```python
from build123d import *

# Parameters (mm, degrees)
F1_DEPTH = 127
F3_D     = 6.7564
F5_D     = 6.7564


with BuildPart() as f1:
    # F0 (on Front) → F1 (new body)
    with BuildSketch(Plane.XZ):
        Polygon((0, 38.1), (0, 0), (15.875, 0), (15.875, 3.175), (3.175, 3.175), (3.175, 38.1), align=None)
    extrude(amount=F1_DEPTH)

    # F3 (through all)
    with Locations(Plane.YZ.offset(3.175)):
        with Locations((-114.3, 25.4), (-63.5, 25.4), (-12.7, 25.4)):
            Hole(F3_D / 2)

    # F5 (through all)
    with Locations(Plane.XY.offset(3.175)):
        with Locations((9.525, -101.6), (9.525, -25.4), (9.525, -76.2), (9.525, -50.8)):
            Hole(F5_D / 2)


solid = f1.part
```
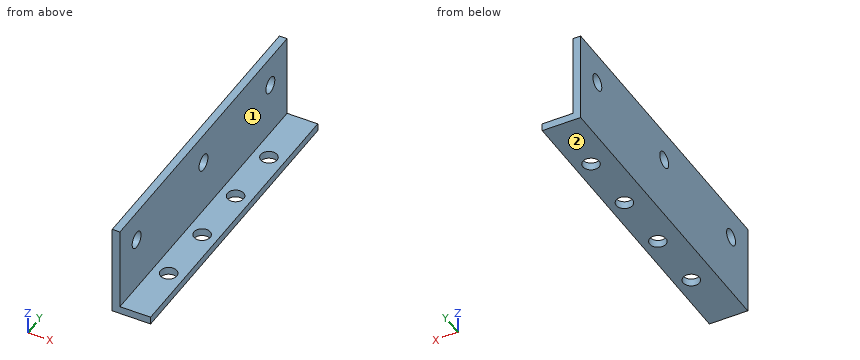
Here's how the part is built. I have some questions about the finished solid (model axes, mm). Face numbers are marked on the shaded views. A direction names the side the tool comes from. Round coordinates to 2 decimals unless told otherwise and drop trailing zeros. Write each loop counter-clockwise with the first axis right and the second up, starting at its lowest first coordinate (ties: lowest second). Pieces come first, ordered by that corner, then holes. Notation, with made-up numbers: M 57,-3.75 L 73,-3.75 A22 ccw 73,15.25 Z; hole C 4.25,-6 d10. An arc over 180 degrees is marked long. Answer as CSV lines item,"result". Start each with the question number.
1. Suppose I cut it at B-B on x = 9. Write out the boundary of the cut face in (y, z) (3 decimals).
2. I need wall thicknesses on probe 1 along Y at (x, z) = (1, 27); probe 2 along Y at (x, z) = (9, 2); probe 3 along Z at (x, y) = (2.1, -114.3). Which ranges of each line are inside material? Lowest first, please.
3. Suppose I cut it at A-A on y = -101.6. Write out the boundary of the cut face in (x, z) (3 decimals).
4. On a 3-axis mill with a long thin cutter (end or side, diameter ignored), from which of +Z, -Z, +X, -X, +Y, -Y can I reach the whole of each face in a straight line? I mean the marked faces 1 and 2. Say none if no direction works.
5. Suppose I cut it at D-D on z = 10.5. Write out the boundary of the cut face in (x, y) (3 decimals).
6. I'm going to push flat-ended pins straight in: pin 1 Ø1.5 at (x, y) = (5, -108.5) entering from +Z (3 decimals); pin 2 Ø9 at (y, z) = (-114.3, 25.4) entering from +X (3 decimals). Where does each tip first touch, or does it pass through?
7. Suppose I cut it at C-C on y = -87. Write out the boundary of the cut face in (x, z) (3 decimals), then the cut area to 3 significant figures.
Check result:
1,outline,"M -127,0 L -104.937,0 L -104.937,3.175 L -127,3.175 Z; M -98.263,0 L -79.537,0 L -79.537,3.175 L -98.263,3.175 Z; M -72.863,0 L -54.137,0 L -54.137,3.175 L -72.863,3.175 Z; M -47.463,0 L -28.737,0 L -28.737,3.175 L -47.463,3.175 Z; M -22.063,0 L 0,0 L 0,3.175 L -22.063,3.175 Z"
2,probe 1,"y = -127 to -117.28, -111.32 to -66.48, -60.52 to -15.68, -9.72 to 0"
2,probe 2,"y = -127 to -104.94, -98.26 to -79.54, -72.86 to -54.14, -47.46 to -28.74, -22.06 to 0"
2,probe 3,"z = 0 to 22.02, 28.78 to 38.1"
3,outline,"M 0,0 L 6.147,0 L 6.147,3.175 L 3.175,3.175 L 3.175,38.1 L 0,38.1 Z; M 12.903,0 L 15.875,0 L 15.875,3.175 L 12.903,3.175 Z"
4,face 1,"+Z, +X, +Y, -Y"
4,face 2,"-Z, +X, -X, +Y, -Y"
5,outline,"M 0,-127 L 3.175,-127 L 3.175,0 L 0,0 Z"
6,pin 1,"stops at z = 3.175"
6,pin 2,"stops at x = 3.175"
7,outline,"M 0,0 L 15.875,0 L 15.875,3.175 L 3.175,3.175 L 3.175,38.1 L 0,38.1 Z"
7,area,"161 mm2"
